```python
from build123d import *

# Parameters (mm, degrees)
F1_DEPTH = 12.7
F3_DEPTH = 12.7
F5_DEPTH = 12.7
F6_R     = 6.35
F7_DEPTH = 12.7


with BuildPart() as f1:
    # F0 (on Right) → F1 (new body)
    with BuildSketch(Plane.YZ):
        with BuildLine():
            ThreePointArc((25.4, 38.1), (12.7, 50.8), (0, 38.1))
            Line((0, 38.1), (25.4, 38.1))
        make_face()
        with BuildLine():
            Line((25.4, 38.1), (0, 38.1))
            ThreePointArc((0, 38.1), (12.7, 25.4), (25.4, 38.1))
        make_face()
        with BuildLine():
            Line((0, 38.1), (0, 0))
            Line((0, 0), (25.4, 0))
            Line((25.4, 0), (25.4, 38.1))
            ThreePointArc((25.4, 38.1), (12.7, 25.4), (0, 38.1))
        make_face()
    extrude(amount=F1_DEPTH)

    # F2 (on face) → F3 (cut)
    with BuildSketch(Plane.YZ.offset(12.7)):
        with BuildLine():
            Line((19.05, 49.098523), (6.35, 49.098523))
            Line((6.35, 49.098523), (6.35, 36.398523))
            ThreePointArc((6.35, 36.398523), (12.7, 42.748523), (19.05, 36.398523))
            Line((19.05, 36.398523), (19.05, 49.098523))
        make_face()
        with BuildLine():
            ThreePointArc((19.05, 36.398523), (12.7, 42.748523), (6.35, 36.398523))
            Line((6.35, 36.398523), (19.05, 36.398523))
        make_face()
        with BuildLine():
            Line((19.05, 36.398523), (6.35, 36.398523))
            ThreePointArc((6.35, 36.398523), (12.7, 30.048523), (19.05, 36.398523))
        make_face()
        with BuildLine():
            ThreePointArc((19.05, 49.098523), (12.7, 50.8), (6.35, 49.098523))
            Line((6.35, 49.098523), (19.05, 49.098523))
        make_face()
    extrude(amount=-F3_DEPTH, mode=Mode.SUBTRACT)

    # F4 (on Top) → F5 (join)
    with BuildSketch(Plane.XY):
        with BuildLine():
            Line((44.45, 25.4), (44.45, 0))
            ThreePointArc((44.45, 0), (53.430256, 3.719744), (57.15, 12.7))
            ThreePointArc((57.15, 12.7), (53.430256, 21.680256), (44.45, 25.4))
        make_face()
        with BuildLine():
            ThreePointArc((44.45, 25.4), (31.75, 12.7), (44.45, 0))
            Line((44.45, 0), (44.45, 25.4))
        make_face()
        with BuildLine():
            Line((12.7, 25.4), (12.7, 0))
            Line((12.7, 0), (44.45, 0))
            ThreePointArc((44.45, 0), (31.75, 12.7), (44.45, 25.4))
            Line((44.45, 25.4), (12.7, 25.4))
        make_face()
    extrude(amount=F5_DEPTH)

    # F6 (on face) → F7 (cut)
    with BuildSketch(Plane.XY.offset(12.7)):
        with Locations((44.45, 12.7)):
            Circle(F6_R)
        with Locations((25.4, 12.7)):
            Circle(F6_R)
    extrude(amount=-F7_DEPTH, mode=Mode.SUBTRACT)


solid = f1.part
```
The listing builds one solid part. Answer for the finished solid, in the listing's coordinates (mm). A direction names the side the tool comes from. Round coordinates to 2 decimals unless told otherwise and drop trailing zeros. Loops run counter-clockwise (first coordinate to the right, second up) from the corner with the lowest first, then second, coordinate; pieces in that order, holes last.
Q1. Given pin 1 Ø7.5 at (y, z) = (10, 33) entering from +X; pin 2 Ø4 at (x, z) = (7.5, 42.5) entering from -Y; pin 3 Ø8 at (x, y) = (42, 17) entering from +Z, each flat-ended and moving along its own axis, determine where each tip first touches the part or whether it passes through.
Q2. Which of the six approach directions +Z, -Z, +X, -X, +Y, -Y give full straight-line access (tool end or side, diameter ignored) to faces 4 (the face through (6.261, 23.745, 44.369)), 5 (the face through (6, 6.35, 43)), 6 (the face through (12.7, 13, 27))?
Q3. Section C-C, the plane z = 7.5 is taken. Determine the outline of the cut face in (x, y), then the cut area to 3 significant figures.
Q4. Find the intervals of material crossed by line 1 (X direction, y = 22.5, z = 13); line 2 (X direction, y = 14, z = 12), in increasing order.
Q5. Section B-B, the plane y = 16.25 is taken. Determine the outline of the cut face in (x, z).
Q6. Section D-D, the plane x = 23.5 is taken. Determine the outline of the cut face in (y, z), then the cut area to 3 significant figures.
Q7. For a pull along Y with two mould halves and no side action, classify faces 1 (the face through (28, 19, 0)), 2 (the face through (6, 19.05, 43)), 3 (the face through (17, 0, 10)) as released by +Y, released by -Y, zero draft, split by the parting line, or undercut.
Q8. Section A-A, the plane x = 4.5 is taken. Determine the outline of the cut face in (y, z).
Completed:
1. pin 1: stops at x = 12.7
1. pin 2: stops at y = 0.23
1. pin 3: stops at z = 12.7
2. face 4: +Z, +X, -X, +Y
2. face 5: +Z, +X, -X
2. face 6: +Z, +X, +Y, -Y
3. outline: (0, 0) - (44.45, 0) arc R12.7 ccw to (44.45, 25.4) - (0, 25.4) - close; hole circle Ø12.7 at (25.4, 12.7); hole circle Ø12.7 at (44.45, 12.7)
3. area: 1,130 mm2
4. line 1: x = 0 to 12.7
4. line 2: x = 0 to 19.18, 31.62 to 38.23, 50.67 to 57.08
5. outline: (0, 0) - (20.14, 0) - (20.14, 12.7) - (12.7, 12.7) - (12.7, 31.13) - (0, 31.13) - close; (30.66, 0) - (39.19, 0) - (39.19, 12.7) - (30.66, 12.7) - close; (49.71, 0) - (56.64, 0) - (56.64, 12.7) - (49.71, 12.7) - close
6. outline: (0, 0) - (6.64, 0) - (6.64, 12.7) - (0, 12.7) - close; (18.76, 0) - (25.4, 0) - (25.4, 12.7) - (18.76, 12.7) - close
6. area: 169 mm2
7. face 1: zero draft
7. face 2: undercut
7. face 3: released by -Y
8. outline: (0, 0) - (25.4, 0) - (25.4, 38.1) arc R12.7 ccw to (19.05, 49.1) - (19.05, 36.4) arc R6.35 cw to (6.35, 36.4) - (6.35, 49.1) arc R12.7 ccw to (0, 38.1) - close
